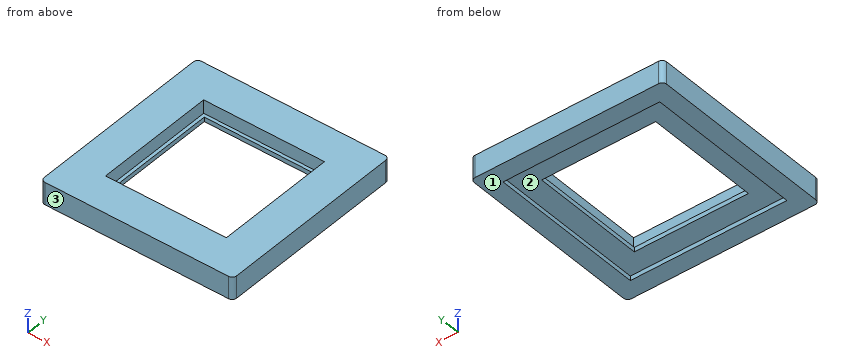
```python
from build123d import *

# Parameters (mm, degrees)
PAD_DEPTH       = 10
SKETCH001_W     = 70
SKETCH001_H     = 70
POCKET_DEPTH    = 2
SKETCH002_W     = 51
SKETCH002_H     = 51
POCKET001_DEPTH = 2
SKETCH003_W     = 54
SKETCH003_H     = 54
POCKET002_DEPTH = 6.001


with BuildPart() as part:
    # Sketch → Pad (new body)
    with BuildSketch(Plane.XY):
        with BuildLine():
            Line((-41, 43), (41, 43))
            ThreePointArc((43, 41), (42.414214, 42.414214), (41, 43))
            Line((43, 41), (43, -41))
            ThreePointArc((41, -43), (42.414214, -42.414214), (43, -41))
            Line((41, -43), (-41, -43))
            ThreePointArc((-43, -41), (-42.414214, -42.414214), (-41, -43))
            Line((-43, -41), (-43, 41))
            ThreePointArc((-41, 43), (-42.414214, 42.414214), (-43, 41))
        make_face()
    extrude(amount=PAD_DEPTH)

    # Sketch001 (on Face9 of Pad) → Pocket (cut)
    with BuildSketch(Plane(origin=(0, 0, 0), x_dir=(1, 0, 0), z_dir=(0, 0, -1))):
        Rectangle(SKETCH001_W, SKETCH001_H)
    extrude(amount=-POCKET_DEPTH, mode=Mode.SUBTRACT)

    # Sketch002 (on Face15 of Pocket) → Pocket001 (cut)
    with BuildSketch(Plane(origin=(0, 0, 2), x_dir=(1, 0, 0), z_dir=(0, 0, -1))):
        Rectangle(SKETCH002_W, SKETCH002_H)
    extrude(amount=-POCKET001_DEPTH, mode=Mode.SUBTRACT)

    # Sketch003 (on Face20 of Pocket001) → Pocket002 (cut, through all)
    with BuildSketch(Plane(origin=(0, 0, 4), x_dir=(1, 0, 0), z_dir=(0, 0, -1))):
        Rectangle(SKETCH003_W, SKETCH003_H)
    extrude(amount=-POCKET002_DEPTH, mode=Mode.SUBTRACT)


solid = part.part
```
Geometry: final body of the model. Coordinates: model frame, mm. Face numbers are marked on the shaded views. Round coordinates to 2 decimals unless told otherwise and drop trailing zeros. Order: outer loops, then holes, each group sorted by start corner. A loop starts at its lowest first (then second) coordinate and runs counter-clockwise, first axis right, second up. Notation, with made-up numbers: (-29, 28) -> (-16, 28) arc R20 cw to (-16, 36) -> close; hole circle Ø6 at (47, 17). An arc over 180 degrees is marked (long way). Use CSV: the item, a comma, the result in double quotes. Start each with the question number.
1) Section A-A (y = 1). Return the cut outline in (x, z).
2) Draft query along Y for the marked faces 1, 2 and 3. Return one class per face: +Y half, -Y half, draft (parallel to the pull), parting line (faces both ways), or undercut.
3) Section B-B (z = 7.75). Return the cut outline in (x, y).
4) First-contact query: pin 1 Ø1.5 at (x, y) = (14.5, 27.5) entering from -Z. Flat tip, straight axial feed; report the tip coordinate or a pass-through.
5) Material intervals for line 1 along X through (y, z) = (-21, 9.25); line 2 along X through (y, z) = (3, 0.5), sorted ascending. Write a range as from..to.
6) Section D-D (y = -33.5). Return the cut outline in (x, z), and give its area (3 significant figures).
Returned:
1,outline,"(-43, 0) -> (-35, 0) -> (-35, 2) -> (-25.5, 2) -> (-25.5, 4) -> (-27, 4) -> (-27, 10) -> (-43, 10) -> close; (25.5, 2) -> (35, 2) -> (35, 0) -> (43, 0) -> (43, 10) -> (27, 10) -> (27, 4) -> (25.5, 4) -> close"
2,face 1,"draft"
2,face 2,"undercut"
2,face 3,"-Y half"
3,outline,"(-43, -41) arc R2 ccw to (-41, -43) -> (41, -43) arc R2 ccw to (43, -41) -> (43, 41) arc R2 ccw to (41, 43) -> (-41, 43) arc R2 ccw to (-43, 41) -> close; hole (-27, -27) -> (27, -27) -> (27, 27) -> (-27, 27) -> close"
4,pin 1,"stops at z = 2"
5,line 1,"x = -43..-27, 27..43"
5,line 2,"x = -43..-35, 35..43"
6,outline,"(-43, 0) -> (-35, 0) -> (-35, 2) -> (35, 2) -> (35, 0) -> (43, 0) -> (43, 10) -> (-43, 10) -> close"
6,area,"720 mm²"
